Answer from the drawing. Dimensions are ordinates in mm from the lowest x, y and z of the part. Coordinates: 2 decimals unless noted, no trailing zeros. Write each loop counter-clockwise with the first axis right and the second up, starting at its lowest first coordinate (ties: lowest second). Pieces come first, ordered by that corner, then holes.
(1) Straight lines are drawn through the part: line 1 along Z through (x, y) = (129.36, 0.85); line 2 along X through (y, z) = (1.3, 18). For each, find the intervals that lie inside material, in ascending order.
(2) The part is cut by section B-B, the plane x = 8. Determine the outline of the cut face in (y, z).
(3) The part is cut by section A-A, the plane z = 52. Determine the outline of the cut face in (x, y), and give its area (3 significant figures).
(4) Determine the mould class of the marked faces 1 and 2 for opening direction Y: pulls with the +Y half, pulls with the -Y half, needs draft (parallel to the pull), parting line crosses it, or undercut.
(5) Given pin 1 (1.8 mm diameter, centred on x = 8, z = 17, fed in from +Y), flat-ended and moving along its own axis, determine where the tip first touches the part or whether it passes through.
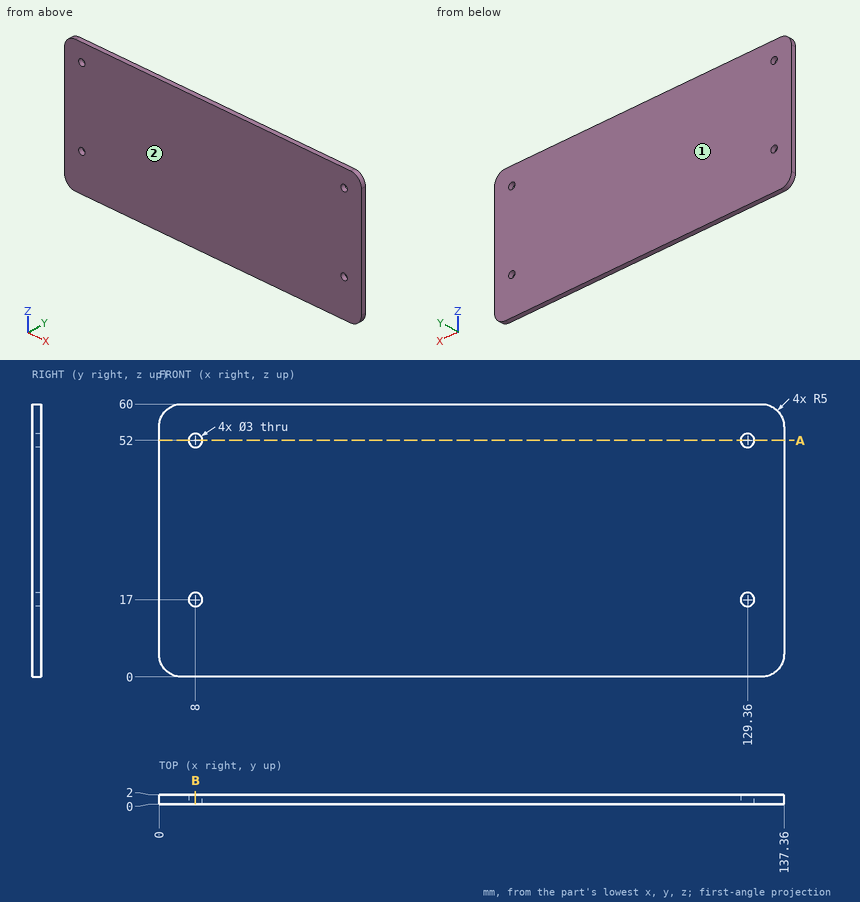
Computed:
1. line 1: z = 0 to 15.5, 18.5 to 50.5, 53.5 to 60
1. line 2: x = 0 to 6.88, 9.12 to 128.24, 130.48 to 137.36
2. outline: (0, 0) - (2, 0) - (2, 15.5) - (0, 15.5) - close; (0, 18.5) - (2, 18.5) - (2, 50.5) - (0, 50.5) - close; (0, 53.5) - (2, 53.5) - (2, 60) - (0, 60) - close
3. outline: (0, 0) - (6.5, 0) - (6.5, 2) - (0, 2) - close; (9.5, 0) - (127.86, 0) - (127.86, 2) - (9.5, 2) - close; (130.86, 0) - (137.36, 0) - (137.36, 2) - (130.86, 2) - close
3. area: 263 mm2
4. face 1: pulls with the +Y half
4. face 2: pulls with the -Y half
5. pin 1: passes through
